```python
from build123d import *

# Parameters (mm, degrees)
F0_R     = 11
F0_R_2   = 7.7
F1_DEPTH = 25
F2_R     = 11
F3_DEPTH = 38
F5_DEPTH = 5
F6_R     = 3.15
F7_DEPTH = 50
F8_SIZE  = 0.8
F9_SIZE  = 0.4
F10_SIZE = 0.4


with BuildPart() as f1:
    # F0 (on Top) → F1 (new body)
    with BuildSketch(Plane.XY):
        Circle(F0_R)
        Circle(F0_R_2, mode=Mode.SUBTRACT)
    extrude(amount=F1_DEPTH)

    # F2 (on face) → F3 (join)
    with BuildSketch(Plane.XY.offset(25)):
        Circle(F2_R)
    extrude(amount=F3_DEPTH)

    # F4 (on face) → F5 (cut)
    with BuildSketch(Plane(origin=(0, 0, 25), x_dir=(1, 0, 0), z_dir=(0, 0, -1))):
        Polygon((-2.915619, -5.05), (2.915619, -5.05), (5.831238, 0), (2.915619, 5.05), (-2.915619, 5.05), (-5.831238, 0), align=None)
    extrude(amount=-F5_DEPTH, mode=Mode.SUBTRACT)

    # F6 (on face) → F7 (cut)
    with BuildSketch(Plane(origin=(0, 0, 30), x_dir=(1, 0, 0), z_dir=(0, 0, -1))):
        Circle(F6_R)
    extrude(amount=-F7_DEPTH, mode=Mode.SUBTRACT)

    # F8
    f8_edges = [f1.edges().sort_by_distance(p)[0] for p in [
        (-11, 0, 0),
        (-11, 0, 63),
    ]]
    chamfer(f8_edges, length=F8_SIZE)

    # F9
    f9_edges = [f1.edges().sort_by_distance(p)[0] for p in [
        (-3.15, 0, 63),
    ]]
    chamfer(f9_edges, length=F9_SIZE)

    # F10
    f10_edges = [f1.edges().sort_by_distance(p)[0] for p in [
        (-7.7, 0, 0),
    ]]
    chamfer(f10_edges, length=F10_SIZE)


solid = f1.part
```
Read the model definition and answer for the solid it produces. Units are mm, in the model's axes. A direction names the side the tool comes from. Give positions to 0.01 mm unless a question says otherwise; leave off trailing zeros. Order: outer loops, then holes, each group sorted by start corner. A loop starts at its lowest first (then second) coordinate and runs counter-clockwise, first axis right, second up.
(1) Given pin 1 (8 mm diameter, centred on x = 7.5, z = 19.5, fed in from +Y); pin 2 (5 mm diameter, centred on x = 0, y = 0, fed in from +Z); pin 3 (3 mm diameter, centred on x = 2.5, y = -0.5, fed in from -Z); pin 4 (4 mm diameter, centred on y = -4, z = 38, fed in from +X), each flat-ended and moving along its own axis, determine where each tip first touches the part or whether it passes through.
(2) For a pull along Y with two mould halves and no side action, classify faces 1 (the flat face through (3, 8, 0)), 2 (the cylindrical face through (-2.38, -10.74, 31.07)), 3 (the flat face through (4.394, -2.49, 27.465)) as released by +Y, released by -Y, zero draft, split by the parting line, or undercut.
(3) Straight lines are drawn through the part: L1, parallel to Y at x = 0, z = 17.5; L2, parallel to Y at x = 0, z = 30.5; L3, parallel to X at y = -3.25, z = 19. For each, find the intervals that lie inside material, in ascending order.
(4) Find section A-A (x = 0). Give the vertices of the cut face in (y, z).
(5) For faces 4 (the cylindrical face through (-1.669, -7.517, 12.528)), 5 (the cylindrical face through (-2.5, 1.917, 46.072)), determine the directions among +Z, -Z, +X, -X, +Y, -Y from which every point of the face is accessible in a straight line to the end or side of a thin tool.
(6) Find section B-B (z = 26.5). Give the vertices of the cut face in (x, y).
Result sheet:
1. pin 1: stops at y = 10.43
1. pin 2: passes through
1. pin 3: stops at z = 30
1. pin 4: stops at x = 10.82
2. face 1: zero draft
2. face 2: split by the parting line
2. face 3: undercut
3. L1: y = -11 to -7.7, 7.7 to 11
3. L2: y = -11 to -3.15, 3.15 to 11
3. L3: x = -10.51 to -6.98, 6.98 to 10.51
4. outline: (-11, 0.8) - (-10.2, 0) - (-8.1, 0) - (-7.7, 0.4) - (-7.7, 25) - (-5.05, 25) - (-5.05, 30) - (-3.15, 30) - (-3.15, 62.6) - (-3.55, 63) - (-10.2, 63) - (-11, 62.2) - close; (3.15, 30) - (5.05, 30) - (5.05, 25) - (7.7, 25) - (7.7, 0.4) - (8.1, 0) - (10.2, 0) - (11, 0.8) - (11, 62.2) - (10.2, 63) - (3.55, 63) - (3.15, 62.6) - close
5. face 4: -Z
5. face 5: +Z, -Z
6. outline: circle Ø22 at (0, 0); hole (-5.83, 0) - (-2.92, -5.05) - (2.92, -5.05) - (5.83, 0) - (2.92, 5.05) - (-2.92, 5.05) - close
